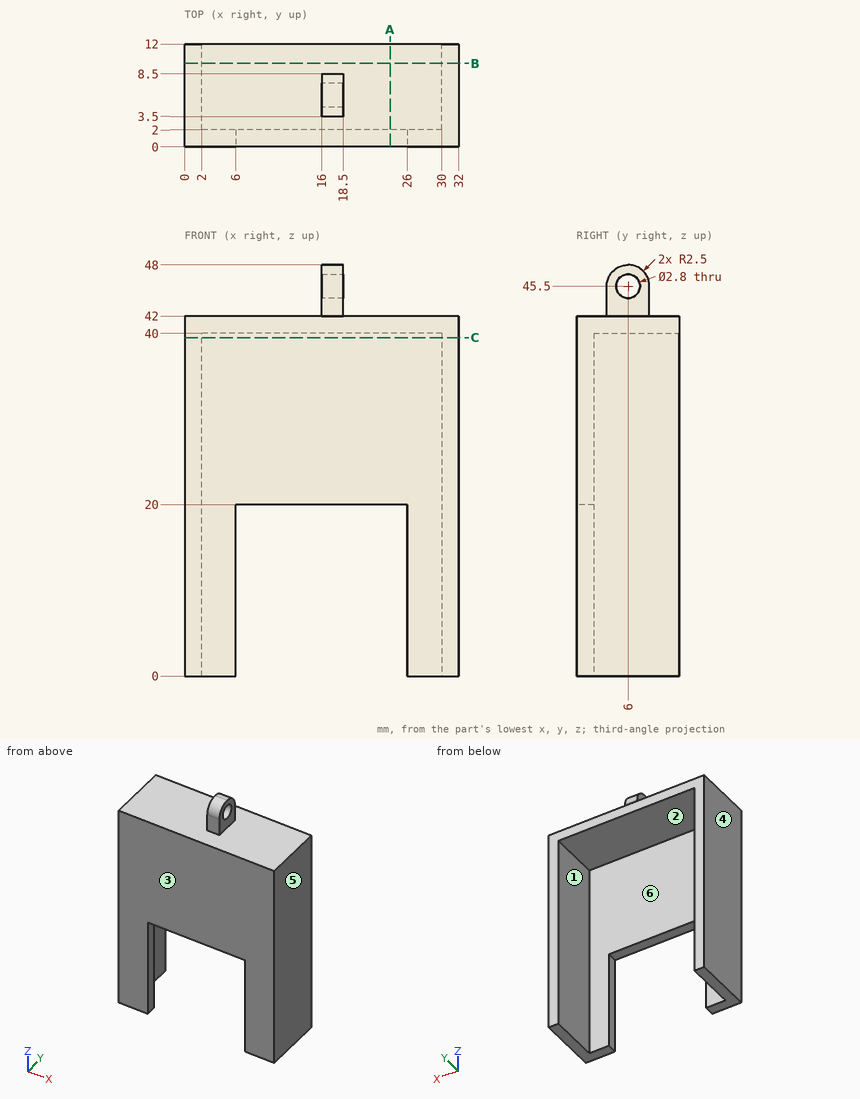
The figure shows three views and two pictorial views of one solid part (mm, origin at its lowest corner). Answer the questions. A direction names the side the tool comes from. Round coordinates to 2 decimals unless told otherwise and drop trailing zeros. Write each loop counter-clockwise with the first axis right and the second up, starting at its lowest first coordinate (ties: lowest second). Pieces come first, ordered by that corner, then holes. Notation, with made-up numbers: M -29,40.5 L 5,40.5 A16 cw 5,63.5 Z; hole C 77.5,83 d11. An arc over 180 degrees is marked long. Use a Markdown table: item, result.
1) Determine the mould class of the marked faces 1, 2, 3 and 4 for opening direction X: pulls with the +X half, pulls with the -X half, needs draft (parallel to the pull), parting line crosses it, or undercut.
Taken from the geometry:
| item | result |
|---|---|
| face 1 | undercut |
| face 2 | undercut |
| face 3 | needs draft |
| face 4 | pulls with the -X half |
2) The part is cut by section A-A on x = 24. Give the vertices of the cut face in (y, z), plus the area to 3 significant figures.
Taken from the geometry:
| item | result |
|---|---|
| outline | M 0,20 L 2,20 L 2,40 L 12,40 L 12,42 L 0,42 Z |
| area | 64.0 mm2 |
3) Consider line 1 (Z direction, x = 16.5, y = 6); line 2 (Y direction, x = 17, z = 45.5); line 3 (X direction, y = 7, z = 31). Determine where each line is inside the solid, lowest interval first. Write a range as [from, to].
Taken from the geometry:
| item | result |
|---|---|
| line 1 | z = [40, 44.1], [46.9, 48] |
| line 2 | y = [3.5, 4.6], [7.4, 8.5] |
| line 3 | x = [0, 2], [30, 32] |
4) Flat-ended cylindrical pins translate along their axes: pin 1 (3 mm diameter, centred on y = 8, z = 14, fed in from -X); pin 2 (2 mm diameter, centred on x = 17, z = 43.5, fed in from +Y); pin 3 (0.6 mm diameter, centred on x = 15.5, y = 1.5, fed in from -Z); pin 4 (3 mm diameter, centred on x = 17.5, y = 9, fed in from -Z). Find the tip coordinate at first contact, or state that the pin passes through.
Taken from the geometry:
| item | result |
|---|---|
| pin 1 | stops at x = 0 |
| pin 2 | stops at y = 8.5 |
| pin 3 | stops at z = 20 |
| pin 4 | stops at z = 40 |
5) The part is cut by section B-B on y = 9.75. Give the vertices of the cut face in (x, z).
Taken from the geometry:
| item | result |
|---|---|
| outline | M 0,0 L 2,0 L 2,40 L 30,40 L 30,0 L 32,0 L 32,42 L 0,42 Z |
6) Which of the six approach directions +Z, -Z, +X, -X, +Y, -Y give full straight-line access (tool end or side, diameter ignored) to the marked faces 5 and 6?
Taken from the geometry:
| item | result |
|---|---|
| face 5 | +Z, -Z, +X, +Y, -Y |
| face 6 | -Z, +Y |
7) The part is cut by section C-C on z = 39.5. Give the vertices of the cut face in (x, y).
Taken from the geometry:
| item | result |
|---|---|
| outline | M 0,0 L 32,0 L 32,12 L 30,12 L 30,2 L 2,2 L 2,12 L 0,12 Z |
